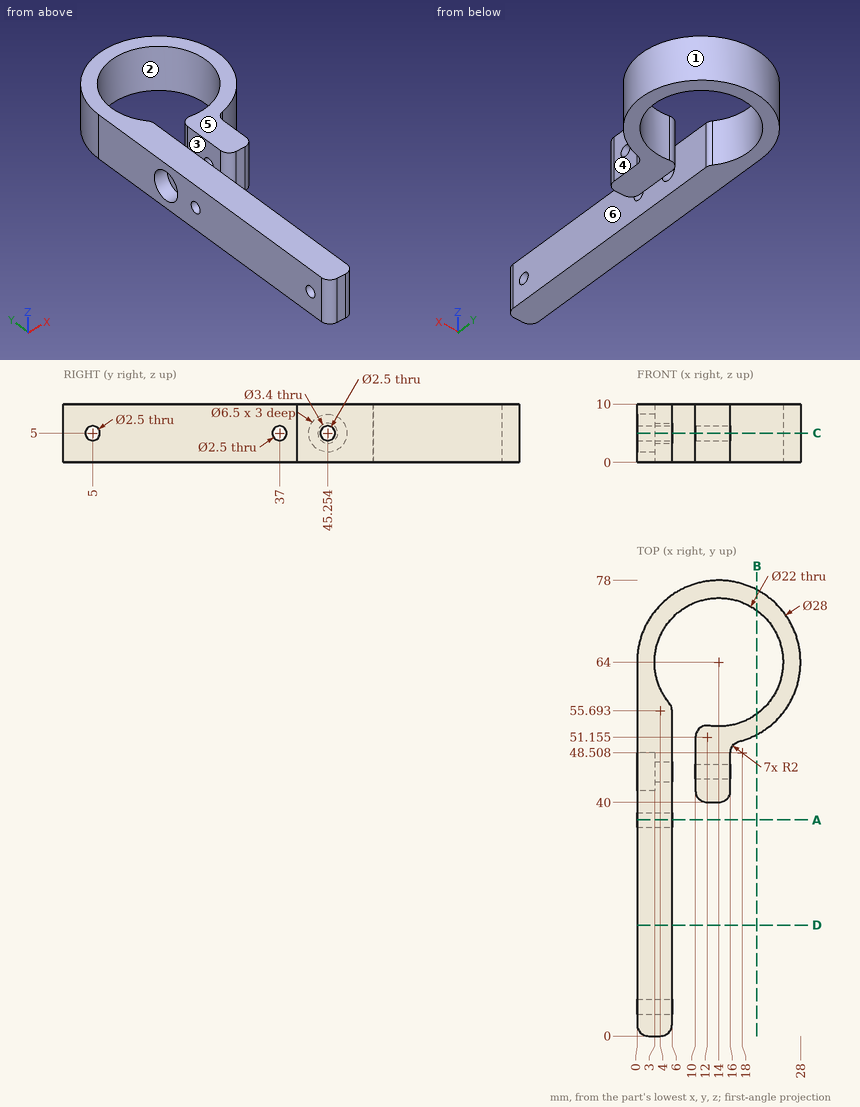
Verification items for this drawing (mm, ordinates from the low corner). A direction names the side the tool comes from. Round coordinates to 2 decimals unless told otherwise and drop trailing zeros. Order: outer loops, then holes, each group sorted by start corner. A loop starts at its lowest first (then second) coordinate and runs counter-clockwise, first axis right, second up.
1) Material ranges on line 1 (Y direction, x = 14.55, z = 5) (1 decimal); line 2 (Y direction, x = 13.05, z = 5); line 3 (X direction, y = 63.5, z = 3.25), recorded low to high.
Geometry says:
line 1: y = 40.1 to 44, 46.5 to 53, 75 to 78
line 2: y = 40 to 44, 46.5 to 53.04, 74.96 to 77.97
line 3: x = 0 to 3.01, 24.99 to 27.99
2) Cross-section at A-A, the plane y = 37. Record the cut outline in (x, z).
Geometry says:
outline: (0, 0) - (6, 0) - (6, 3.75) - (0, 3.75) - close; (0, 6.25) - (6, 6.25) - (6, 10) - (0, 10) - close
3) Depth check by flat-ended pin: pin 1 (2 mm diameter, centred on y = 46.5, z = 3, fed in from +X); pin 2 (2.5 mm diameter, centred on y = 44.5, z = 3.5, fed in from -X); pin 3 (1.6 mm diameter, centred on x = 13, z = 7, fed in from -Y); pin 4 (3 mm diameter, centred on x = 7, y = 26.5, fed in from -Z). Enter the tip coordinate at first touch or a pass-through.
Geometry says:
pin 1: stops at x = 16
pin 2: stops at x = 3
pin 3: stops at y = 40
pin 4: stops at z = 0
4) Cross-section at D-D, the plane y = 19. Record the cut outline in (x, z), plus the area to 3 significant figures.
Geometry says:
outline: (0, 0) - (6, 0) - (6, 10) - (0, 10) - close
area: 60.0 mm2
5) Tool access check on the marked faces 5 and 6. Record the directions out of +Z, -Z, +X, -X, +Y, -Y that give a thin tool (end or side, any length) a straight path to the whole face; none if there is none.
Geometry says:
face 5: +Z, +X, -X, +Y, -Y
face 6: +Z, -Z, -Y
6) Cross-section at C-C, the plane z = 5. Give the number of separate pieces and of enclosed holes in the cut face, plus the area to 3 significant figures.
Geometry says:
separate pieces: 5
enclosed holes: 0
area: 539 mm2
7) Draft check along X on the marked faces 1, 2, 3 and 4. Enter one of: +X half, -X half, draft (parallel to the pull), parting line (faces both ways), or undercut.
Geometry says:
face 1: parting line
face 2: undercut
face 3: undercut
face 4: +X half
8) Cross-section at B-B, the plane x = 20.5. Record the cut outline in (y, z).
Geometry says:
outline: (51.6, 0) - (55.13, 0) - (55.13, 10) - (51.6, 10) - close; (72.87, 0) - (76.4, 0) - (76.4, 10) - (72.87, 10) - close
